Verification items for the finished model (mm, model axes). Face numbers are marked on the shaded views. Coordinates: 2 decimals unless noted, no trailing zeros. Write each loop counter-clockwise with the first axis right and the second up, starting at its lowest first coordinate (ties: lowest second). Pieces come first, ordered by that corner, then holes. Notation, with made-up numbers: (16, -15) -> (45, -15) arc R16 ccw to (45, -4) -> close; hole circle Ø4 at (42, -35.5). An arc over 180 degrees is marked (long way). Use CSV: the item, a comma, the result in double quotes.
Autodesk Inventor part; units mm, degrees
ref_plane "YZ Plane" through (0, 0, 0) normal (1, 0, 0) x (0, 1, 0)
ref_plane "XZ Plane" through (0, 0, 0) normal (0, 1, 0) x (-1, 0, 0)
ref_plane "XY Plane" through (0, 0, 0) normal (0, 0, 1) x (1, 0, 0)
sketch "Эскиз1" plane through (0, 0, 0) normal (0, 1, 0) x (-1, 0, 0)
  circle A0 centre (0, 0) radius 48
  line L0 (31, 15.207) -> (-31, 15.207)
  line L1 (-31, 15.207) -> (-31, -15.207)
  line L2 (-31, -15.207) -> (31, -15.207)
  line L3 (31, -15.207) -> (31, 15.207)
  circle A1 centre (31, 15.207) radius 1.5
  circle A2 centre (31, -15.207) radius 1.5
  circle A3 centre (-31, 15.207) radius 1.5
  circle A4 centre (-31, -15.207) radius 1.5
  dimension "d0" = 96
  dimension "d1" = 62
  dimension "d2" = 30.414
  dimension "d3" = 31
  dimension "d4" = 15.207
  dimension "d5" = 3
  dimension "d6" = 3
  dimension "d7" = 3
  dimension "d8" = 3
extrude "Выдавливание1" add sketch "Эскиз1" along normal blind 3 contours A0 | L0 A1 L3 A2 L2 A4 L1 A3
sketch "Эскиз2" plane through (0, 3, 0) normal (0, 1, 0) x (1, 0, 0)
  circle A0 centre (0, 0) radius 27.25
  circle A1 centre (-22.15, 0) radius 3
  circle A2 centre (22.15, 0) radius 3
  circle A3 centre (0, 15.543) radius 3
  dimension "d11" = 54.5
  dimension "d12" = 6
  dimension "d13" = 6
  dimension "d14" = 44.3
  dimension "d15" = 22.15
  dimension "d16" = 6
  dimension "d17" = 15.543
extrude "Выдавливание2" add sketch "Эскиз2" along normal blind 13 contours A1 | A2 | A3
sketch "Эскиз3" plane through (0, 16, -15.543) normal (0, 1, 0) x (-1, 0, 0)
  circle A0 centre (0, 0) radius 2
  circle A1 centre (-22.15, 15.543) radius 2.2
  circle A2 centre (22.15, 15.543) radius 2
  circle A3 centre (22.15, 15.543) radius 3
  circle A4 centre (22.15, 15.543) radius 3
  circle A5 centre (0, 0) radius 3
  circle A6 centre (0, 0) radius 3
  circle A7 centre (-22.15, 15.543) radius 3
  circle A8 centre (-22.15, 15.543) radius 3
  point P0 (0, 15.543)
  dimension "d20" = 4
  dimension "d21" = 4.4
  dimension "d22" = 4
  dimension "d23" = 6
  dimension "d24" = 6
  dimension "d25" = 6
extrude "Выдавливание3" cut sketch "Эскиз3" against normal blind 5 contours A0 | A1 | A2
properties part number "openmv"
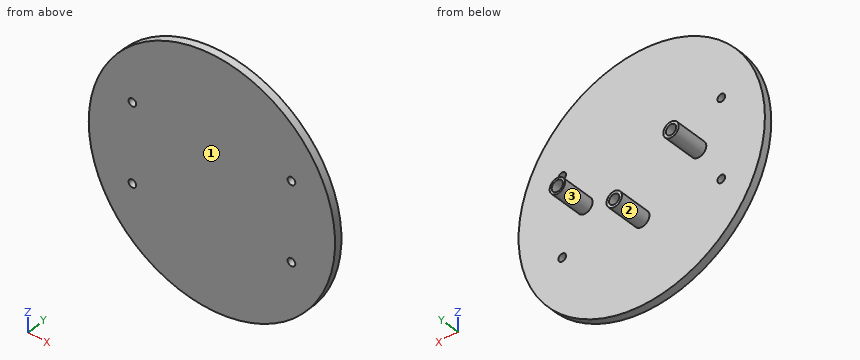
1) Cross-section at C-C (x = -31). Record the boundary of the cut face in (y, z), plus the area to 3 significant figures.
Return value:
outline,"(0, -36.65) -> (3, -36.65) -> (3, -16.71) -> (0, -16.71) -> close; (0, -13.71) -> (3, -13.71) -> (3, 13.71) -> (0, 13.71) -> close; (0, 16.71) -> (3, 16.71) -> (3, 36.65) -> (0, 36.65) -> close"
area,"202 mm2"
2) Gauge pin test, flat ends, axial feed: pin 1 (3 mm diameter, centred on x = 11.5, y = 2, fed in from -Z); pin 2 (4 mm diameter, centred on y = 13, z = -15, fed in from +X); pin 3 (4 mm diameter, centred on x = -37.5, y = 4, fed in from +Z). Record the tip position at first contact, or that the pin passes through.
Return value:
pin 1,"z = -46.95"
pin 2,"x = 3"
pin 3,"z = 32.01"
3) Cross-section at B-B (z = 0). Record the boundary of the cut face in (x, y), plus the area to 3 significant figures.
Return value:
outline,"(-48, 0) -> (48, 0) -> (48, 3) -> (25.15, 3) -> (25.15, 16) -> (24.35, 16) -> (24.35, 11) -> (19.95, 11) -> (19.95, 16) -> (19.15, 16) -> (19.15, 3) -> (-19.15, 3) -> (-19.15, 16) -> (-20.15, 16) -> (-20.15, 11) -> (-24.15, 11) -> (-24.15, 16) -> (-25.15, 16) -> (-25.15, 3) -> (-48, 3) -> close"
area,"402 mm2"
4) Cross-section at A-A (y = 12.25). Record the boundary of the cut face in (x, z).
Return value:
outline,"circle Ø6 at (-22.15, 0); circle Ø6 at (0, -15.54); circle Ø6 at (22.15, 0); hole circle Ø4 at (-22.15, 0); hole circle Ø4 at (0, -15.54); hole circle Ø4.4 at (22.15, 0)"
5) Scan lines: L1, parallel to Z at x = 0, y = 14.5; L2, parallel to Y at x = 16, z = -26.5; L3, parallel to Z at x = 22.15, y = 14.2. Record each from-to range of solid material in increasing order.
Return value:
L1,"-18.54 to -17.54, -13.54 to -12.54"
L2,"0 to 3"
L3,"-3 to -2.2, 2.2 to 3"
6) Cross-section at D-D (x = 22.15). Record the boundary of the cut face in (y, z).
Return value:
outline,"(0, -42.58) -> (3, -42.58) -> (3, -3) -> (16, -3) -> (16, -2.2) -> (11, -2.2) -> (11, 2.2) -> (16, 2.2) -> (16, 3) -> (3, 3) -> (3, 42.58) -> (0, 42.58) -> close"
7) Mould release check, pull along X, two halves, no side actions. Record for the marked faces 1, 2 and 3: released by +X, released by -X, zero draft, split by the parting line, or undercut.
Return value:
face 1,"zero draft"
face 2,"split by the parting line"
face 3,"undercut"
